Autodesk Inventor part; units mm, degrees
ref_plane "ip_st_1_1_XY" through (1.25, 3.25, 0) normal (1, 0, 0) x (0, 0, -1)
ref_plane "ip_st_1_1_YZ" through (1.25, 3.25, 0) normal (0, 0, -1) x (0, 1, 0)
ref_plane "ip_st_1_1_ZX" through (1.25, 3.25, 0) normal (0, 1, 0) x (1, 0, 0)
sketch "Sketch_1" plane through (0, 0, 0) normal (0, 0, 1) x (1, 0, 0)
  line L0 (2.5, 0) -> (0, 0)
  arc A0 (0, 2.6) -> (0.1, 2.5) centre (0.1, 2.6) ccw
  line L1 (0.1, 2.5) -> (2.4, 2.5)
  arc A1 (2.4, 2.5) -> (2.5, 2.6) centre (2.4, 2.6) ccw
  line L2 (2.5, 2.6) -> (2.5, 2.9)
  line L3 (2.5, 2.9) -> (1.5328, 2.9)
  arc A2 (0.9672, 2.9) -> (1.5328, 2.9) centre (1.25, 3.25) ccw
  line L4 (0.9672, 2.9) -> (0, 2.9)
  line L5 (0, 2.9) -> (0, 2.6)
revolve "Revolution1" add sketch "Sketch_1" angle 360 about axis through (2.5, 0, 0) along (1, 0, 0)
ref_plane "ip_st_1_1_XY" through (1.25, 3.25, 0) normal (1, 0, 0) x (0, 0, -1)
ref_plane "ip_st_1_1_YZ" through (1.25, 3.25, 0) normal (0, 0, -1) x (0, 1, 0)
ref_plane "ip_st_1_1_ZX" through (1.25, 3.25, 0) normal (0, 1, 0) x (1, 0, 0)
ref_plane "ip_st_1_10_XY" through (1.25, -3.1947, -0.5972) normal (1, 0, 0) x (0, 0, -1)
ref_plane "ip_st_1_10_YZ" through (1.25, -3.1947, -0.5972) normal (0, 0, -1) x (0, 1, 0)
ref_plane "ip_st_1_10_ZX" through (1.25, -3.1947, -0.5972) normal (0, 1, 0) x (1, 0, 0)
ref_plane "ip_st_1_11_XY" through (1.25, -2.7632, -1.7109) normal (1, 0, 0) x (0, 0, -1)
ref_plane "ip_st_1_11_YZ" through (1.25, -2.7632, -1.7109) normal (0, 0, -1) x (0, 1, 0)
ref_plane "ip_st_1_11_ZX" through (1.25, -2.7632, -1.7109) normal (0, 1, 0) x (1, 0, 0)
ref_plane "ip_st_1_12_XY" through (1.25, -1.9586, -2.5936) normal (1, 0, 0) x (0, 0, -1)
ref_plane "ip_st_1_12_YZ" through (1.25, -1.9586, -2.5936) normal (0, 0, -1) x (0, 1, 0)
ref_plane "ip_st_1_12_ZX" through (1.25, -1.9586, -2.5936) normal (0, 1, 0) x (1, 0, 0)
ref_plane "ip_st_1_13_XY" through (1.25, -0.8894, -3.1259) normal (1, 0, 0) x (0, 0, -1)
ref_plane "ip_st_1_13_YZ" through (1.25, -0.8894, -3.1259) normal (0, 0, -1) x (0, 1, 0)
ref_plane "ip_st_1_13_ZX" through (1.25, -0.8894, -3.1259) normal (0, 1, 0) x (1, 0, 0)
ref_plane "ip_st_1_14_XY" through (1.25, 0.2999, -3.2361) normal (1, 0, 0) x (0, 0, -1)
ref_plane "ip_st_1_14_YZ" through (1.25, 0.2999, -3.2361) normal (0, 0, -1) x (0, 1, 0)
ref_plane "ip_st_1_14_ZX" through (1.25, 0.2999, -3.2361) normal (0, 1, 0) x (1, 0, 0)
ref_plane "ip_st_1_15_XY" through (1.25, 1.4486, -2.9093) normal (1, 0, 0) x (0, 0, -1)
ref_plane "ip_st_1_15_YZ" through (1.25, 1.4486, -2.9093) normal (0, 0, -1) x (0, 1, 0)
ref_plane "ip_st_1_15_ZX" through (1.25, 1.4486, -2.9093) normal (0, 1, 0) x (1, 0, 0)
ref_plane "ip_st_1_16_XY" through (1.25, 2.4018, -2.1895) normal (1, 0, 0) x (0, 0, -1)
ref_plane "ip_st_1_16_YZ" through (1.25, 2.4018, -2.1895) normal (0, 0, -1) x (0, 1, 0)
ref_plane "ip_st_1_16_ZX" through (1.25, 2.4018, -2.1895) normal (0, 1, 0) x (1, 0, 0)
ref_plane "ip_st_1_17_XY" through (1.25, 3.0305, -1.174) normal (1, 0, 0) x (0, 0, -1)
ref_plane "ip_st_1_17_YZ" through (1.25, 3.0305, -1.174) normal (0, 0, -1) x (0, 1, 0)
ref_plane "ip_st_1_17_ZX" through (1.25, 3.0305, -1.174) normal (0, 1, 0) x (1, 0, 0)
ref_plane "ip_st_1_2_XY" through (1.25, 3.0305, 1.174) normal (1, 0, 0) x (0, 0, -1)
ref_plane "ip_st_1_2_YZ" through (1.25, 3.0305, 1.174) normal (0, 0, -1) x (0, 1, 0)
ref_plane "ip_st_1_2_ZX" through (1.25, 3.0305, 1.174) normal (0, 1, 0) x (1, 0, 0)
ref_plane "ip_st_1_3_XY" through (1.25, 2.4018, 2.1895) normal (1, 0, 0) x (0, 0, -1)
ref_plane "ip_st_1_3_YZ" through (1.25, 2.4018, 2.1895) normal (0, 0, -1) x (0, 1, 0)
ref_plane "ip_st_1_3_ZX" through (1.25, 2.4018, 2.1895) normal (0, 1, 0) x (1, 0, 0)
ref_plane "ip_st_1_4_XY" through (1.25, 1.4486, 2.9093) normal (1, 0, 0) x (0, 0, -1)
ref_plane "ip_st_1_4_YZ" through (1.25, 1.4486, 2.9093) normal (0, 0, -1) x (0, 1, 0)
ref_plane "ip_st_1_4_ZX" through (1.25, 1.4486, 2.9093) normal (0, 1, 0) x (1, 0, 0)
ref_plane "ip_st_1_5_XY" through (1.25, 0.2999, 3.2361) normal (1, 0, 0) x (0, 0, -1)
ref_plane "ip_st_1_5_YZ" through (1.25, 0.2999, 3.2361) normal (0, 0, -1) x (0, 1, 0)
ref_plane "ip_st_1_5_ZX" through (1.25, 0.2999, 3.2361) normal (0, 1, 0) x (1, 0, 0)
ref_plane "ip_st_1_6_XY" through (1.25, -0.8894, 3.1259) normal (1, 0, 0) x (0, 0, -1)
ref_plane "ip_st_1_6_YZ" through (1.25, -0.8894, 3.1259) normal (0, 0, -1) x (0, 1, 0)
ref_plane "ip_st_1_6_ZX" through (1.25, -0.8894, 3.1259) normal (0, 1, 0) x (1, 0, 0)
ref_plane "ip_st_1_7_XY" through (1.25, -1.9586, 2.5936) normal (1, 0, 0) x (0, 0, -1)
ref_plane "ip_st_1_7_YZ" through (1.25, -1.9586, 2.5936) normal (0, 0, -1) x (0, 1, 0)
ref_plane "ip_st_1_7_ZX" through (1.25, -1.9586, 2.5936) normal (0, 1, 0) x (1, 0, 0)
ref_plane "ip_st_1_8_XY" through (1.25, -2.7632, 1.7109) normal (1, 0, 0) x (0, 0, -1)
ref_plane "ip_st_1_8_YZ" through (1.25, -2.7632, 1.7109) normal (0, 0, -1) x (0, 1, 0)
ref_plane "ip_st_1_8_ZX" through (1.25, -2.7632, 1.7109) normal (0, 1, 0) x (1, 0, 0)
ref_plane "ip_st_1_9_XY" through (1.25, -3.1947, 0.5972) normal (1, 0, 0) x (0, 0, -1)
ref_plane "ip_st_1_9_YZ" through (1.25, -3.1947, 0.5972) normal (0, 0, -1) x (0, 1, 0)
ref_plane "ip_st_1_9_ZX" through (1.25, -3.1947, 0.5972) normal (0, 1, 0) x (1, 0, 0)
ref_plane "ip_st_1a_XY" through (0, 0, 0) normal (1, 0, 0) x (0, 0, -1)
ref_plane "ip_st_1a_YZ" through (0, 0, 0) normal (0, 0, -1) x (0, 1, 0)
ref_plane "ip_st_1a_ZX" through (0, 0, 0) normal (0, 1, 0) x (1, 0, 0)
ref_plane "ip_st_2a_XY" through (0.1562, 0, 0) normal (1, 0, 0) x (0, 0, -1)
ref_plane "ip_st_2a_YZ" through (0.1562, 0, 0) normal (0, 0, -1) x (0, 1, 0)
ref_plane "ip_st_2a_ZX" through (0.1562, 0, 0) normal (0, 1, 0) x (1, 0, 0)
properties part number "MF85ZZ Inner Ring" material "ステンレス鋼 440C"
Geometry: final body of the model. Coordinates: model frame, mm. Coordinates: 2 decimals unless noted, no trailing zeros. Order: outer loops, then holes, each group sorted by start corner. A loop starts at its lowest first (then second) coordinate and runs counter-clockwise, first axis right, second up. Notation, with made-up numbers: (53, -5) - (85, -5) arc R20 cw to (85, 15) - close; hole circle Ø1 at (50.25, -36.75). An arc over 180 degrees is marked (long way). Use one line per item in the form item = value.
1) Section A-A (z = 0). Return loops of the section in (x, y), then the cut area to 3 significant figures.
Solutions:
outline = (0, -2.9) - (0.97, -2.9) arc R0.45 cw to (1.53, -2.9) - (2.5, -2.9) - (2.5, -2.6) arc R0.1 ccw to (2.4, -2.5) - (0.1, -2.5) arc R0.1 ccw to (0, -2.6) - close; (0, 2.6) arc R0.1 ccw to (0.1, 2.5) - (2.4, 2.5) arc R0.1 ccw to (2.5, 2.6) - (2.5, 2.9) - (1.53, 2.9) arc R0.45 cw to (0.97, 2.9) - (0, 2.9) - close
area = 1.91 mm^2
2) Ray query, L1, parallel to Z at x = 0.95, y = 0; L2, parallel to X at y = 1.8, z = -1.85; L3, parallel to Z at x = 2.15, y = -1.25. Return the intervals inside material, ascending.
Solutions:
L1 = -2.9 to -2.5, 2.5 to 2.9
L2 = 0 to 2.5
L3 = -2.62 to -2.17, 2.17 to 2.62
3) Section D-D (x = 1.3). Return loops of the section in (y, z).
Solutions:
outline = circle Ø5.61 at (0, 0); hole circle Ø5 at (0, 0)
4) Section C-C (x = 0.85). Return loops of the section in (y, z), then the cut area to 3 significant figures.
Solutions:
outline = circle Ø5.8 at (0, 0); hole circle Ø5 at (0, 0)
area = 6.79 mm^2
5) Mould query, pull axis Y, two halves, no side actions, for faces 1 (the face through (0.5, -2.9, -0.1)), 2 (the face through (1.27, -0.54, -2.44)). Classes: +Y half, -Y half, draft (parallel to the pull), parting line (faces both ways), or undercut.
Solutions:
face_1 = parting line
face_2 = undercut
